Verification items for this drawing (mm, ordinates from the low corner). A direction names the side the tool comes from. Round coordinates to 2 decimals unless told otherwise and drop trailing zeros. Write each loop counter-clockwise with the first axis right and the second up, starting at its lowest first coordinate (ties: lowest second). Pieces come first, ordered by that corner, then holes. Notation, with made-up numbers: (-37.75, 86) -> (0.25, 86) arc R18 cw to (0.25, 121) -> close; hole circle Ø1 at (77, 78.5). An arc over 180 degrees is marked (long way). One line per question, with ' | ' between items.
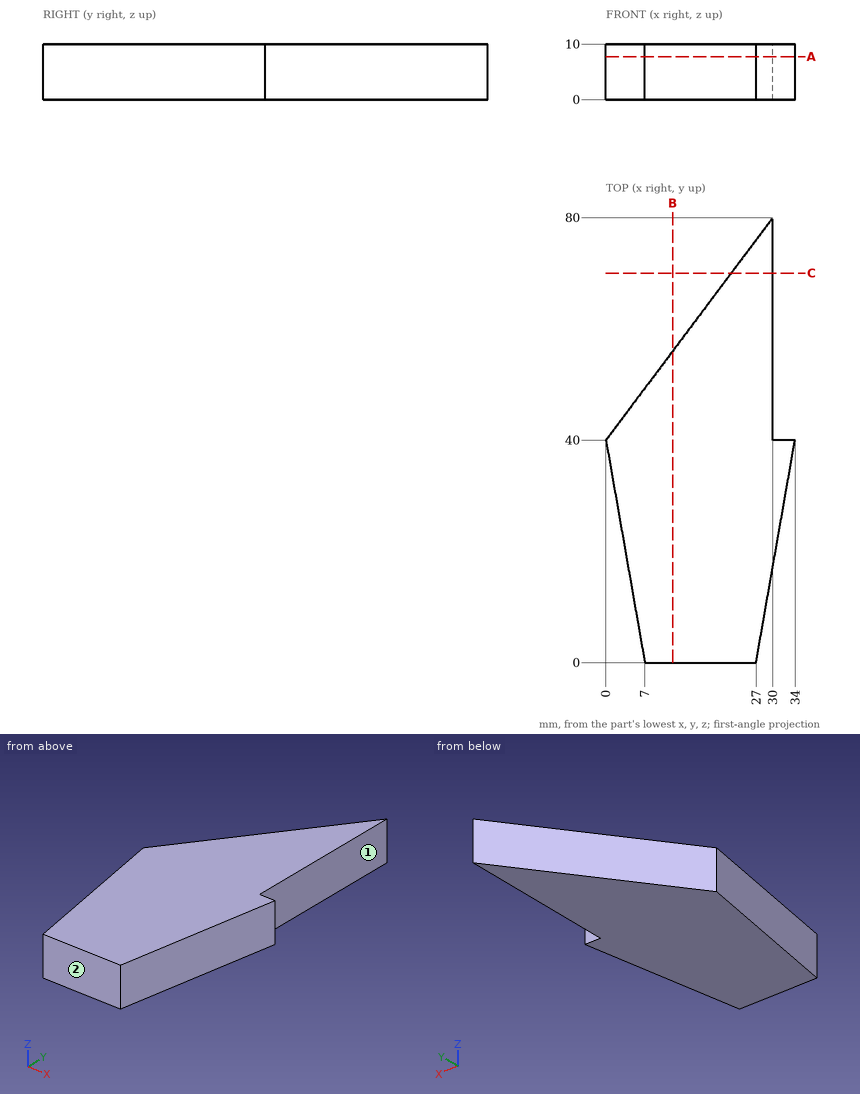
(1) Access from +Z, -Z, +X, -X, +Y, -Y to the whole of each face (thin tool, end or side, straight path). Record for the marked faces 1 and 2.
Resolved:
face 1: +Z, -Z, +X, +Y | face 2: +Z, -Z, +X, -X, -Y
(2) Material ranges on line 1 (X direction, y = 33, z = 0.5) (3 decimals); line 2 (Y direction, x = 16.5, z = 5.75); line 3 (X direction, y = 28.5, z = 8), recorded low to high.
Resolved:
line 1: x = 1.225 to 32.775 | line 2: y = 0 to 62 | line 3: x = 2.01 to 31.99
(3) Sectioned sample at B-B on x = 12. Record the cut outline in (y, z), then the cut area to 3 significant figures.
Resolved:
outline: (0, 0) -> (56, 0) -> (56, 10) -> (0, 10) -> close | area: 560 mm2
(4) Go/stop test with flat-tipped pins: pin 1 (2 mm diameter, centred on x = 4, z = 7.5, fed in from +Y); pin 2 (1 mm diameter, centred on x = 15.5, z = 9, fed in from +Y); pin 3 (2 mm diameter, centred on x = 28, z = 7.5, fed in from +Y). Record where each tip stops, or that it passes through.
Resolved:
pin 1: stops at y = 46.67 | pin 2: stops at y = 61.33 | pin 3: stops at y = 78.67
(5) Sectioned sample at C-C on y = 70. Record the cut outline in (x, z).
Resolved:
outline: (22.5, 0) -> (30, 0) -> (30, 10) -> (22.5, 10) -> close
(6) Sectioned sample at A-A on z = 7.75. Record the cut outline in (x, y), then the cut area to 3 significant figures.
Resolved:
outline: (0, 40) -> (7, 0) -> (27, 0) -> (34, 40) -> (30, 40) -> (30, 80) -> close | area: 1,680 mm2
